```python
from build123d import *

# Parameters (mm, degrees)
SKETCH_1_W          = 10
SKETCH_1_H          = 10
SKETCH_1_W_2        = 8
SKETCH_1_H_2        = 8
EXTRUDE_1_DEPTH     = 210
CUT_EXTRUDE_3_DEPTH = 10
SKETCH_5_R          = 2.5
CUT_EXTRUDE_4_DEPTH = 10
SKETCH_11_R         = 2.125
CUT_EXTRUDE_6_DEPTH = 10


with BuildPart() as part:
    # 草图1 → 凸台-拉伸1 (new body)
    with BuildSketch(Plane(origin=(0, 0, 0), x_dir=(1, 0, 0), z_dir=(0, 1, 0))):
        Rectangle(SKETCH_1_W, SKETCH_1_H)
        Rectangle(SKETCH_1_W_2, SKETCH_1_H_2, mode=Mode.SUBTRACT)
    extrude(amount=EXTRUDE_1_DEPTH)

    # 草图4 → 切除-拉伸3 (cut)
    with BuildSketch(Plane(origin=(0, 0, -5), x_dir=(-1, 0, 0), z_dir=(0, 0, -1))):
        Polygon((-5, 210), (5, 200), (5, 210), align=None)
        Polygon((5, 0), (-5, 0), (5, 10), align=None)
    extrude(amount=-CUT_EXTRUDE_3_DEPTH, mode=Mode.SUBTRACT)

    # 草图5 → 切除-拉伸4 (cut)
    with BuildSketch(Plane.ZY.offset(5)):
        with Locations((0, 165)):
            Circle(SKETCH_5_R)
        with Locations(Location((0, 45, 0), (0, 0, 180))):
            Circle(SKETCH_5_R)
        with Locations((0, 195)):
            Circle(SKETCH_5_R)
        with Locations(Location((0, 15, 0), (0, 0, 180))):
            Circle(SKETCH_5_R)
    extrude(amount=-CUT_EXTRUDE_4_DEPTH, mode=Mode.SUBTRACT)

    # 草图11 → 切除-拉伸6 (cut)
    with BuildSketch(Plane.XY.offset(5)):
        with Locations((0, 130)):
            Circle(SKETCH_11_R)
        with Locations(Location((0, 80, 0), (0, 0, 180))):
            Circle(SKETCH_11_R)
    extrude(amount=-CUT_EXTRUDE_6_DEPTH, mode=Mode.SUBTRACT)


solid = part.part
```
Design review of the part built by this model. Coordinates are the model's own, in mm. A direction names the side the tool comes from. Give positions to 0.01 mm unless a question says otherwise; leave off trailing zeros. Order: outer loops, then holes, each group sorted by start corner. A loop starts at its lowest first (then second) coordinate and runs counter-clockwise, first axis right, second up. Notation, with made-up numbers: M 87,83 L 104,83 A17 ccw 104,107 Z; hole C 5.5,73 d4. An arc over 180 degrees is marked long. One line per question, with ' | ' between items. Start each with the question number.
Q1. We need section C-C (y = 64.5). Write out the cut boundary in (x, z), plus the area to 3 significant figures.
Q2. Machinability: for faces 4 (the face through (0, 104, 4)), 5 (the face through (-5, 104, 0)), which of the approach directions +Z, -Z, +X, -X, +Y, -Y give a long, thin tool a straight path to every point of the face, cutting with its end or side? Answer none if there is none.
Q3. We need section D-D (z = -0.75). State how many separate pieces and enclosed holes the cut face has, plus the area to 3 significant figures.
Q4. We need section B-B (x = 0). Write out the cut boundary in (y, z) (3 decimals), plus the area to 3 significant figures.
Q5. For L1, parallel to X at y = 145.5, z = 0.25; L2, parallel to Z at x = 4.65, y = 15, list the stretches that pass through material, from the lowest coordinate up. Write a range as [from, to].
Q6. The part is to be moulded in two halves that separate along Z. For faces 1 (the face through (0.277, 77.893, -4.493)), 2 (the face through (-4.51, 167.48, -0.33)), 3 (the face through (0, 104, 5)), say which applies: +Z half, -Z half, draft (parallel to the pull), parting line (faces both ways), or undercut.
Q7. We need section A-A (y = 195). Write out the cut boundary in (x, z), plus the area to 3 significant figures.
Returned:
1) outline: M -5,-5 L 5,-5 L 5,5 L -5,5 Z; hole M -4,-4 L 4,-4 L 4,4 L -4,4 Z | area: 36.0 mm2
2) face 4: +Y, -Y | face 5: +Z, -Z, -X, +Y, -Y
3) separate pieces: 10 | enclosed holes: 0 | area: 362 mm2
4) outline: M 5,-5 L 77.875,-5 L 77.875,-4 L 5,-4 Z; M 5,4 L 77.875,4 L 77.875,5 L 5,5 Z; M 82.125,-5 L 127.875,-5 L 127.875,-4 L 82.125,-4 Z; M 82.125,4 L 127.875,4 L 127.875,5 L 82.125,5 Z; M 132.125,-5 L 205,-5 L 205,-4 L 132.125,-4 Z; M 132.125,4 L 205,4 L 205,5 L 132.125,5 Z | area: 383 mm2
5) L1: [-5, -4], [4, 5] | L2: [-5, -2.5], [2.5, 5]
6) face 1: draft | face 2: undercut | face 3: +Z half
7) outline: M -5,-5 L 5,-5 L 5,-2.5 L 4,-2.5 L 4,-4 L -4,-4 L -4,-2.5 L -5,-2.5 Z; M -5,2.5 L -4,2.5 L -4,4 L 4,4 L 4,2.5 L 5,2.5 L 5,5 L -5,5 Z | area: 26.0 mm2
